For this review, take the finished solid that the model builds, in its own axes (mm). A direction names the side the tool comes from. Give positions to 0.01 mm unless a question says otherwise; leave off trailing zeros. Write each loop counter-clockwise with the first axis right and the second up, starting at its lowest first coordinate (ties: lowest second). Pieces come first, ordered by that corner, then holes.
Q1. We need section C-C (z = 5.1). Write out the cut boundary in (x, y).
Q2. For line 1 (X direction, y = 75, z = 2.75); line 2 (Y direction, x = -25, z = 4.6); line 3 (X direction, y = 15, z = 1.6), list the stretches that pass through material, from the lowest coordinate up.
Q3. Insertion check: P1, Ø8, axis at x = -25, y = 75, coming from the -Z side. The pin has a flat end and moves straight along its axis. Give the tip position at first contact, or say it passes through.
Q4. Machinability: for faces 4 (the flat face through (-50, -1, 3)), 5 (the flat face through (3.25, -25, 3)), which of the approach directions +Z, -Z, +X, -X, +Y, -Y give a long, thin tool a straight path to every point of the face, cutting with its end or side? Answer none if there is none.
Q5. Mouldability with a two-part tool opening along X and no side actions: class faces 1 (the flat face through (50, -1, 3)), 2 (the cylindrical face through (-20.504, -0.198, 3.042)), 3 (the flat face through (-12, 1, 6)) as released by +X, released by -X, zero draft, split by the parting line, or undercut.
Q6. We need section A-A (x = -25). Write out the cut boundary in (y, z), then the cut area to 3 significant figures.
Q7. We need section D-D (y = -65). Write out the cut boundary in (x, z).
Q8. We need section B-B (y = 0). Write out the cut boundary in (x, z).
```python
from build123d import *

# Parameters (mm, degrees)
F0_W     = 100
F0_H     = 200
F0_W_2   = 6.5
F0_H_2   = 100.5
F1_DEPTH = 6
F2_D     = 9


with BuildPart() as f1:
    # F0 (on Top) → F1 (new body)
    with BuildSketch(Plane.XY):
        Rectangle(F0_W, F0_H)
        with Locations((0, -24.75)):
            Rectangle(F0_W_2, F0_H_2, mode=Mode.SUBTRACT)
    extrude(amount=F1_DEPTH)

    # F2 (through all)
    with Locations(Plane(origin=(0, 0, 0), x_dir=(1, 0, 0), z_dir=(0, 0, -1))):
        with Locations((-25, 75), (25, 75), (-25, 0), (25, 0), (25, -75), (-25, -75)):
            Hole(F2_D / 2)


solid = f1.part
```
Computed:
1. outline: (-50, -100) - (50, -100) - (50, 100) - (-50, 100) - close; hole circle Ø9 at (-25, -75); hole circle Ø9 at (-25, 0); hole circle Ø9 at (-25, 75); hole (-3.25, -75) - (3.25, -75) - (3.25, 25.5) - (-3.25, 25.5) - close; hole circle Ø9 at (25, -75); hole circle Ø9 at (25, 0); hole circle Ø9 at (25, 75)
2. line 1: x = -50 to -29.5, -20.5 to 20.5, 29.5 to 50
2. line 2: y = -100 to -79.5, -70.5 to -4.5, 4.5 to 70.5, 79.5 to 100
2. line 3: x = -50 to -3.25, 3.25 to 50
3. P1: passes through
4. face 4: +Z, -Z, -X, +Y, -Y
4. face 5: +Z, -Z
5. face 1: released by +X
5. face 2: undercut
5. face 3: zero draft
6. outline: (-100, 0) - (-79.5, 0) - (-79.5, 6) - (-100, 6) - close; (-70.5, 0) - (-4.5, 0) - (-4.5, 6) - (-70.5, 6) - close; (4.5, 0) - (70.5, 0) - (70.5, 6) - (4.5, 6) - close; (79.5, 0) - (100, 0) - (100, 6) - (79.5, 6) - close
6. area: 1,040 mm2
7. outline: (-50, 0) - (-3.25, 0) - (-3.25, 6) - (-50, 6) - close; (3.25, 0) - (50, 0) - (50, 6) - (3.25, 6) - close
8. outline: (-50, 0) - (-29.5, 0) - (-29.5, 6) - (-50, 6) - close; (-20.5, 0) - (-3.25, 0) - (-3.25, 6) - (-20.5, 6) - close; (3.25, 0) - (20.5, 0) - (20.5, 6) - (3.25, 6) - close; (29.5, 0) - (50, 0) - (50, 6) - (29.5, 6) - close
